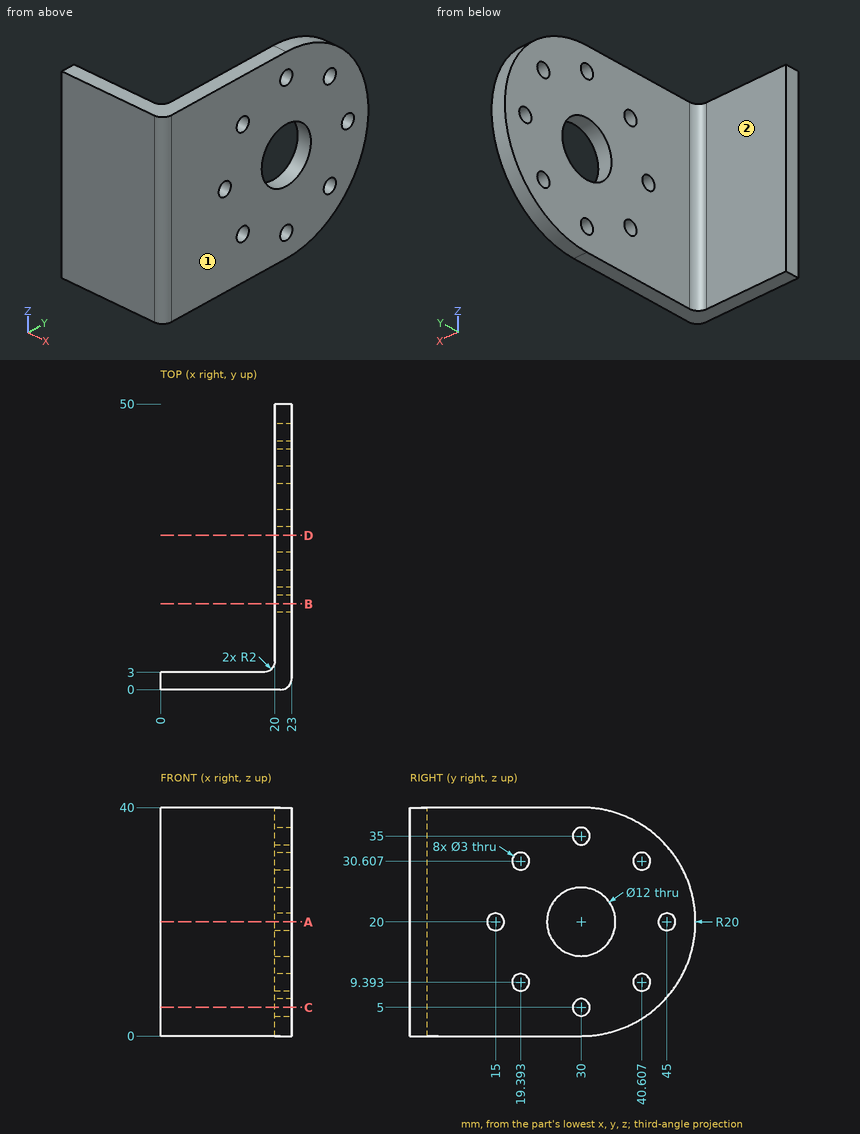
Verification items for this drawing (mm, ordinates from the low corner). A direction names the side the tool comes from. Round coordinates to 2 decimals unless told otherwise and drop trailing zeros. Loops run counter-clockwise (first coordinate to the right, second up) from the corner with the lowest first, then second, coordinate; pieces in that order, holes last. Notation, with made-up numbers: (-10, -14) - (29, -14) arc R12 cw to (29, 3) - close; hole circle Ø9 at (27, 5.25). An arc over 180 degrees is marked (long way). Answer as CSV lines item,"result". Start each with the question number.
Item 1: Set-up check for the marked faces 1 and 2: record each of +Z, -Z, +X, -X, +Y, -Y from which the full face is reachable in a straight line by a thin tool's end or side.
Item 2: Depth check by flat-ended pin: P1, Ø5, axis at y = 19.39, z = 30.61, coming from the -X side; P2, Ø2.5, axis at y = 19.39, z = 9.39, coming from the -X side; P3, Ø10, axis at x = 20, y = 10, coming from the -Z side. Enter the tip coordinate at first touch or a pass-through.
Item 3: Scan lines: line 1 (Y direction, x = 21, z = 20); line 2 (X direction, y = 37.5, z = 27.5); line 3 (Y direction, x = 22.35, z = 20) (1 decimal). Record each from-to range of solid material in increasing order. Write a range as [from, to].
Item 4: Section check A-A (z = 20). Record the boundary of the cut face in (x, y).
Item 5: Section check D-D (y = 27). Record the boundary of the cut face in (x, z).
Item 6: Section check C-C (z = 5). Record the boundary of the cut face in (x, y).
Item 7: Section check B-B (y = 15). Record the boundary of the cut face in (x, z), and give its area (3 significant figures).
Report:
1,face 1,"+Z, -Z, +X, +Y, -Y"
1,face 2,"+Z, -Z, -X, +Y"
2,P1,"stops at x = 20"
2,P2,"passes through"
2,P3,"stops at z = 0"
3,line 1,"y = [0, 13.5], [16.5, 24], [36, 43.5], [46.5, 50]"
3,line 2,"x = [20, 23]"
3,line 3,"y = [0.5, 13.5], [16.5, 24], [36, 43.5], [46.5, 50]"
4,outline,"(0, 0) - (21, 0) arc R2 ccw to (23, 2) - (23, 13.5) - (20, 13.5) - (20, 5) arc R2 cw to (18, 3) - (0, 3) - close; (20, 16.5) - (23, 16.5) - (23, 24) - (20, 24) - close; (20, 36) - (23, 36) - (23, 43.5) - (20, 43.5) - close; (20, 46.5) - (23, 46.5) - (23, 50) - (20, 50) - close"
5,outline,"(20, 0) - (23, 0) - (23, 14.8) - (20, 14.8) - close; (20, 25.2) - (23, 25.2) - (23, 40) - (20, 40) - close"
6,outline,"(0, 0) - (21, 0) arc R2 ccw to (23, 2) - (23, 28.5) - (20, 28.5) - (20, 5) arc R2 cw to (18, 3) - (0, 3) - close; (20, 31.5) - (23, 31.5) - (23, 43.23) - (20, 43.23) - close"
7,outline,"(20, 0) - (23, 0) - (23, 18.5) - (20, 18.5) - close; (20, 21.5) - (23, 21.5) - (23, 40) - (20, 40) - close"
7,area,"111 mm2"
